from build123d import *

# Parameters (mm, degrees)
SKETCH1_W                          = 2.5
SKETCH1_H                          = 4.25
CUT_EXTRUDE1_DEPTH                 = 3.5
CUT_EXTRUDE2_DEPTH                 = 3.5
CUT_EXTRUDE3_DEPTH                 = 3.5
CUT_EXTRUDE4_DEPTH                 = 3.5
CUT_EXTRUDE5_DEPTH                 = 3.5
CUT_EXTRUDE6_DEPTH                 = 3.5
CUT_EXTRUDE7_DEPTH                 = 3.5
CUT_EXTRUDE8_DEPTH                 = 3.5
CUT_EXTRUDE9_DEPTH                 = 3.5
CUT_EXTRUDE10_DEPTH                = 3.5
CUT_EXTRUDE11_DEPTH                = 3.5
CUT_EXTRUDE12_DEPTH                = 3.5
CUT_EXTRUDE13_DEPTH                = 3.5
CUT_EXTRUDE14_DEPTH                = 3.5
CUT_EXTRUDE15_DEPTH                = 3.5
SKETCH17_W                         = 3.8000508
SKETCH17_H                         = 3
F_4_0_4_DIAMETER_HOLE1_D           = 4
F_4_0_4_DIAMETER_HOLE1_DEPTH       = 6.3000508
TAP_DRILL_FOR_M2_5X0_45_TAP1_D     = 2.05
TAP_DRILL_FOR_M2_5X0_45_TAP1_DEPTH = 6


with BuildPart() as part:
    # Sketch1 → Revolve1 (revolve)
    with BuildSketch(Plane(origin=(0, 0, 0), x_dir=(-1, 0, 0), z_dir=(0, 0, -1))):
        with Locations((-1.25, 2.125)):
            Rectangle(SKETCH1_W, SKETCH1_H)
    revolve(axis=Axis((2.5, 0, 0), (-1, 0, 0)))

    # Sketch2 → Cut-Extrude1 (cut, through all)
    with BuildSketch(Plane(origin=(2.5, 0, 0), x_dir=(0, 0, -1), z_dir=(1, 0, 0))):
        with BuildLine():
            ThreePointArc((2.585993953, 3.372704445), (2.472774023, 2.780247912), (2.135335156, 2.280289405))
            ThreePointArc((2.135335156, 2.280289405), (2.321584435, 2.090364014), (2.491001044, 1.88528242))
            ThreePointArc((2.491001044, 1.88528242), (3.023492692, 2.168612866), (3.624538392, 2.219283994))
            ThreePointArc((3.624538392, 2.219283994), (3.158365508, 2.843805077), (2.585993953, 3.372704445))
        make_face()
    extrude(amount=-CUT_EXTRUDE1_DEPTH, mode=Mode.SUBTRACT)

    # Sketch3 → Cut-Extrude2 (cut, through all)
    with BuildSketch(Plane(origin=(2.5, 0, 0), x_dir=(0, 0, -1), z_dir=(1, 0, 0))):
        with BuildLine():
            ThreePointArc((3.734225512, 2.029300328), (3.389820178, 1.534115047), (2.87820299, 1.214628975))
            ThreePointArc((2.87820299, 1.214628975), (2.971100557, 0.96536909), (3.042456131, 0.709109787))
            ThreePointArc((3.042456131, 0.709109787), (3.644152332, 0.751361165), (4.213844705, 0.553184234))
            ThreePointArc((4.213844705, 0.553184234), (4.041990194, 1.313322226), (3.734225512, 2.029300328))
        make_face()
    extrude(amount=-CUT_EXTRUDE2_DEPTH, mode=Mode.SUBTRACT)

    # Sketch4 → Cut-Extrude3 (cut, through all)
    with BuildSketch(Plane(origin=(2.5, 0, 0), x_dir=(0, 0, -1), z_dir=(1, 0, 0))):
        with BuildLine():
            ThreePointArc((4.236775558, 0.335011746), (3.72073563, 0.022719752), (3.12340338, -0.061051839))
            ThreePointArc((3.12340338, -0.061051839), (3.106886401, -0.326546919), (3.067842913, -0.589674367))
            ThreePointArc((3.067842913, -0.589674367), (3.634704928, -0.795807707), (4.074538988, -1.208566106))
            ThreePointArc((4.074538988, -1.208566106), (4.226718055, -0.444245969), (4.236775558, 0.335011746))
        make_face()
    extrude(amount=-CUT_EXTRUDE3_DEPTH, mode=Mode.SUBTRACT)

    # Sketch5 → Cut-Extrude4 (cut, through all)
    with BuildSketch(Plane(origin=(2.5, 0, 0), x_dir=(0, 0, -1), z_dir=(1, 0, 0))):
        with BuildLine():
            ThreePointArc((4.00674862, -1.417203408), (3.40830209, -1.492603993), (2.82853895, -1.326176235))
            ThreePointArc((2.82853895, -1.326176235), (2.705463361, -1.562), (2.562771785, -1.786498468))
            ThreePointArc((2.562771785, -1.786498468), (2.996784021, -2.205374197), (3.230708464, -2.761344386))
            ThreePointArc((3.230708464, -2.761344386), (3.680607966, -2.124999999), (4.00674862, -1.417203408))
        make_face()
    extrude(amount=-CUT_EXTRUDE4_DEPTH, mode=Mode.SUBTRACT)

    # Sketch6 → Cut-Extrude5 (cut, through all)
    with BuildSketch(Plane(origin=(2.5, 0, 0), x_dir=(0, 0, -1), z_dir=(1, 0, 0))):
        with BuildLine():
            ThreePointArc((3.083918444, -2.92437122), (2.506542154, -2.749842949), (2.044594439, -2.361992714))
            ThreePointArc((2.044594439, -2.361992714), (1.836241128, -2.52736909), (1.614574134, -2.674420753))
            ThreePointArc((1.614574134, -2.674420753), (1.840691933, -3.233611452), (1.828259097, -3.836661137))
            ThreePointArc((1.828259097, -3.836661137), (2.498087322, -3.438322226), (3.083918444, -2.92437122))
        make_face()
    extrude(amount=-CUT_EXTRUDE5_DEPTH, mode=Mode.SUBTRACT)

    # Sketch7 → Cut-Extrude6 (cut, through all)
    with BuildSketch(Plane(origin=(2.5, 0, 0), x_dir=(0, 0, -1), z_dir=(1, 0, 0))):
        with BuildLine():
            ThreePointArc((1.627850754, -3.925888679), (1.17137831, -3.531609077), (0.907120976, -2.989399193))
            ThreePointArc((0.907120976, -2.989399193), (0.649516122, -3.055733105), (0.387201946, -3.099911394))
            ThreePointArc((0.387201946, -3.099911394), (0.366327487, -3.702727912), (0.109687121, -4.248584321))
            ThreePointArc((0.109687121, -4.248584321), (0.883624686, -4.157127303), (1.627850754, -3.925888679))
        make_face()
    extrude(amount=-CUT_EXTRUDE6_DEPTH, mode=Mode.SUBTRACT)

    # Sketch8 → Cut-Extrude7 (cut, through all)
    with BuildSketch(Plane(origin=(2.5, 0, 0), x_dir=(0, 0, -1), z_dir=(1, 0, 0))):
        with BuildLine():
            ThreePointArc((-0.109687122, -4.248584322), (-0.366327487, -3.702727912), (-0.387201947, -3.099911394))
            ThreePointArc((-0.387201947, -3.099911394), (-0.649516122, -3.055733105), (-0.907120975, -2.989399193))
            ThreePointArc((-0.907120975, -2.989399193), (-1.171378309, -3.531609077), (-1.627850753, -3.92588868))
            ThreePointArc((-1.627850753, -3.92588868), (-0.883624686, -4.157127304), (-0.109687122, -4.248584322))
        make_face()
    extrude(amount=-CUT_EXTRUDE7_DEPTH, mode=Mode.SUBTRACT)

    # Sketch9 → Cut-Extrude8 (cut, through all)
    with BuildSketch(Plane(origin=(2.5, 0, 0), x_dir=(0, 0, -1), z_dir=(1, 0, 0))):
        with BuildLine():
            ThreePointArc((-1.828259096, -3.836661137), (-1.840691932, -3.233611453), (-1.614574133, -2.674420754))
            ThreePointArc((-1.614574133, -2.674420754), (-1.836241128, -2.527369091), (-2.044594439, -2.361992714))
            ThreePointArc((-2.044594439, -2.361992714), (-2.506542155, -2.749842949), (-3.083918444, -2.92437122))
            ThreePointArc((-3.083918444, -2.92437122), (-2.498087322, -3.438322226), (-1.828259096, -3.836661137))
        make_face()
    extrude(amount=-CUT_EXTRUDE8_DEPTH, mode=Mode.SUBTRACT)

    # Sketch10 → Cut-Extrude9 (cut, through all)
    with BuildSketch(Plane(origin=(2.5, 0, 0), x_dir=(0, 0, -1), z_dir=(1, 0, 0))):
        with BuildLine():
            ThreePointArc((-3.230708464, -2.761344387), (-2.996784021, -2.205374197), (-2.562771785, -1.786498468))
            ThreePointArc((-2.562771785, -1.786498468), (-2.705463361, -1.562), (-2.82853895, -1.326176236))
            ThreePointArc((-2.82853895, -1.326176236), (-3.40830209, -1.492603994), (-4.006748619, -1.417203409))
            ThreePointArc((-4.006748619, -1.417203409), (-3.680607966, -2.125), (-3.230708464, -2.761344387))
        make_face()
    extrude(amount=-CUT_EXTRUDE9_DEPTH, mode=Mode.SUBTRACT)

    # Sketch11 → Cut-Extrude10 (cut, through all)
    with BuildSketch(Plane(origin=(2.5, 0, 0), x_dir=(0, 0, -1), z_dir=(1, 0, 0))):
        with BuildLine():
            ThreePointArc((-4.074538989, -1.208566105), (-3.634704928, -0.795807707), (-3.067842914, -0.589674368))
            ThreePointArc((-3.067842914, -0.589674368), (-3.106886402, -0.326546919), (-3.12340338, -0.061051839))
            ThreePointArc((-3.12340338, -0.061051839), (-3.720735631, 0.022719752), (-4.236775558, 0.335011747))
            ThreePointArc((-4.236775558, 0.335011747), (-4.226718056, -0.444245968), (-4.074538989, -1.208566105))
        make_face()
    extrude(amount=-CUT_EXTRUDE10_DEPTH, mode=Mode.SUBTRACT)

    # Sketch12 → Cut-Extrude11 (cut, through all)
    with BuildSketch(Plane(origin=(2.5, 0, 0), x_dir=(0, 0, -1), z_dir=(1, 0, 0))):
        with BuildLine():
            ThreePointArc((-4.213844706, 0.553184234), (-3.644152332, 0.751361165), (-3.042456131, 0.709109788))
            ThreePointArc((-3.042456131, 0.709109788), (-2.971100557, 0.96536909), (-2.87820299, 1.214628975))
            ThreePointArc((-2.87820299, 1.214628975), (-3.389820179, 1.534115046), (-3.734225513, 2.029300326))
            ThreePointArc((-3.734225513, 2.029300326), (-4.041990195, 1.313322226), (-4.213844706, 0.553184234))
        make_face()
    extrude(amount=-CUT_EXTRUDE11_DEPTH, mode=Mode.SUBTRACT)

    # Sketch13 → Cut-Extrude12 (cut, through all)
    with BuildSketch(Plane(origin=(2.5, 0, 0), x_dir=(0, 0, -1), z_dir=(1, 0, 0))):
        with BuildLine():
            ThreePointArc((-2.585993952, 3.372704446), (-3.158365508, 2.843805077), (-3.624538391, 2.219283994))
            ThreePointArc((-3.624538391, 2.219283994), (-3.023492692, 2.168612865), (-2.491001044, 1.885282419))
            ThreePointArc((-2.491001044, 1.885282419), (-2.321584435, 2.090364014), (-2.135335156, 2.280289405))
            ThreePointArc((-2.135335156, 2.280289405), (-2.472774022, 2.780247912), (-2.585993952, 3.372704446))
        make_face()
    extrude(amount=-CUT_EXTRUDE12_DEPTH, mode=Mode.SUBTRACT)

    # Sketch14 → Cut-Extrude13 (cut, through all)
    with BuildSketch(Plane(origin=(2.5, 0, 0), x_dir=(0, 0, -1), z_dir=(1, 0, 0))):
        with BuildLine():
            ThreePointArc((-0.990620545, 4.132937326), (-1.728630733, 3.882568195), (-2.408516462, 3.501649391))
            ThreePointArc((-2.408516462, 3.501649391), (-1.880043697, 3.210891701), (-1.508829246, 2.735472593))
            ThreePointArc((-1.508829246, 2.735472593), (-1.270645273, 2.85391601), (-1.023248474, 2.951667081))
            ThreePointArc((-1.023248474, 2.951667081), (-1.128162774, 3.545650656), (-0.990620545, 4.132937326))
        make_face()
    extrude(amount=-CUT_EXTRUDE13_DEPTH, mode=Mode.SUBTRACT)

    # Sketch15 → Cut-Extrude14 (cut, through all)
    with BuildSketch(Plane(origin=(2.5, 0, 0), x_dir=(0, 0, -1), z_dir=(1, 0, 0))):
        with BuildLine():
            ThreePointArc((-0.776040155, 4.178547795), (-0.411518069, 3.69797819), (-0.265767165, 3.112674704))
            ThreePointArc((-0.265767165, 3.112674704), (0, 3.124), (0.265767165, 3.112674704))
            ThreePointArc((0.265767165, 3.112674704), (0.411518069, 3.69797819), (0.776040156, 4.178547795))
            ThreePointArc((0.776040156, 4.178547795), (0, 4.25), (-0.776040155, 4.178547795))
        make_face()
    extrude(amount=-CUT_EXTRUDE14_DEPTH, mode=Mode.SUBTRACT)

    # Sketch16 → Cut-Extrude15 (cut, through all)
    with BuildSketch(Plane(origin=(2.5, 0, 0), x_dir=(0, 0, -1), z_dir=(1, 0, 0))):
        with BuildLine():
            ThreePointArc((0.990620545, 4.132937326), (1.128162774, 3.545650656), (1.023248474, 2.951667081))
            ThreePointArc((1.023248474, 2.951667081), (1.270645273, 2.85391601), (1.508829246, 2.735472593))
            ThreePointArc((1.508829246, 2.735472593), (1.880043697, 3.210891701), (2.408516462, 3.50164939))
            ThreePointArc((2.408516462, 3.50164939), (1.728630733, 3.882568195), (0.990620545, 4.132937326))
        make_face()
    extrude(amount=-CUT_EXTRUDE15_DEPTH, mode=Mode.SUBTRACT)

    # Sketch17 → Revolve2 (revolve)
    with BuildSketch(Plane.XY):
        with Locations((-1.9000254, 1.5)):
            Rectangle(SKETCH17_W, SKETCH17_H)
    revolve(axis=Axis((-3.8000508, 0, 0), (1, 0, 0)))

    # Ø4.0 (4) Diameter Hole1
    with Locations(Plane(origin=(2.5, 0, 0), x_dir=(0, 0, -1), z_dir=(1, 0, 0))):
        with Locations((0, 0)):
            Hole(F_4_0_4_DIAMETER_HOLE1_D / 2, depth=F_4_0_4_DIAMETER_HOLE1_DEPTH)

    # Tap Drill for M2.5x0.45 Tap1
    with Locations(Plane(origin=(-1.9000508, 2.999970615, 0.013278053), x_dir=(0, -0.004426018, 0.999990205), z_dir=(0, 0.999990205, 0.004426018))):
        with Locations((0, 0)):
            Hole(TAP_DRILL_FOR_M2_5X0_45_TAP1_D / 2, depth=TAP_DRILL_FOR_M2_5X0_45_TAP1_DEPTH)


solid = part.part
Source: CAD feature listing. Evaluate the final solid. Frame: model axes, mm. A direction names the side the tool comes from. Give positions to 0.01 mm unless a question says otherwise; leave off trailing zeros. Write each loop counter-clockwise with the first axis right and the second up, starting at its lowest first coordinate (ties: lowest second). Pieces come first, ordered by that corner, then holes. Notation, with made-up numbers: M 67.5,82.5 L 110.5,82.5 A22 cw 110.5,91.5 Z; hole C -9.75,53.25 d8. An arc over 180 degrees is marked long. Answer as a JSON object with one key per item and string values.
Q1. Cut plane A-A, the plane y = -3.25. Return the cut outline in (x, z).
Geometry check:
{"outline": "M 0,-1.84 L 2.5,-1.84 L 2.5,-1 L 0,-1 Z; M 0,-0.4 L 2.5,-0.4 L 2.5,0.4 L 0,0.4 Z; M 0,1 L 2.5,1 L 2.5,1.84 L 0,1.84 Z"}
Q2. Cut plane B-B, the plane x = -3.25. Return the cut outline in (y, z), then the cut area to 3 significant figures.
Geometry check:
{"outline": "C 0,0 d6; hole C 0,0 d4", "area": "15.7 mm^2"}
Q3. Cut plane C-C, the plane y = 1. Return the cut outline in (x, z), then the cut area to 3 significant figures.
Geometry check:
{"outline": "M -3.8,-2.83 L 0,-2.83 L 0,-2.96 L 2.5,-2.96 L 2.5,-1.73 L -3.8,-1.73 Z; M -3.8,1.73 L 2.5,1.73 L 2.5,2.96 L 0,2.96 L 0,2.83 L -3.8,2.83 Z", "area": "14.5 mm^2"}
Q4. Cut plane D-D, the plane z = 0. Count the separate pieces of the cut face and the enclosed holes in it, then the cut area to 3 significant figures.
Geometry check:
{"separate pieces": "4", "enclosed holes": "0", "area": "11.9 mm^2"}
Q5. Ray query, line 1 along Y through (x, z) = (0.5, 0); line 2 along Z through (x, y) = (1.5, 1.5); line 3 along Z through (x, y) = (1.5, -0.25). Return the intervals inside material, ascending.
Geometry check:
{"line 1": "y = -4.25 to -2, 2 to 3.12", "line 2": "z = -3.35 to -1.32, 1.32 to 3.35", "line 3": "z = -3.11 to -1.98, 1.98 to 3.11"}
Q6. Mould query, pull axis Z, two halves, no side actions, for faces 1 (the face through (-1.873, 1.384, -2.662)), 2 (the face through (1.268, -2.746, 2.499)), 3 (the face through (1.268, -2.198, -2.992)). Classes: +Z half, -Z half, draft (parallel to the pull), parting line (faces both ways), or undercut.
Geometry check:
{"face 1": "parting line", "face 2": "undercut", "face 3": "-Z half"}
Q7. Access query for faces 4 (the face through (1.268, 3.706, 0.415)), 5 (the face through (1.268, -0.791, -3.627)), 6 (the face through (1.27, -1.49, 3.4)). Directions: +Z, -Z, +X, -X, +Y, -Y. A direction counts if a zero-diameter tool reaches every point of the face in a straight line with its end or side. Return the directions, or none.
Geometry check:
{"face 4": "+X, -X, +Y", "face 5": "-Z, +X, -X", "face 6": "+X, -X"}
